Build history of the part. All positions in model axes, mm. Face numbers are marked on the shaded views. A direction names the side the tool comes from. Coordinates: 2 decimals unless noted, no trailing zeros. Write each loop counter-clockwise with the first axis right and the second up, starting at its lowest first coordinate (ties: lowest second). Pieces come first, ordered by that corner, then holes.
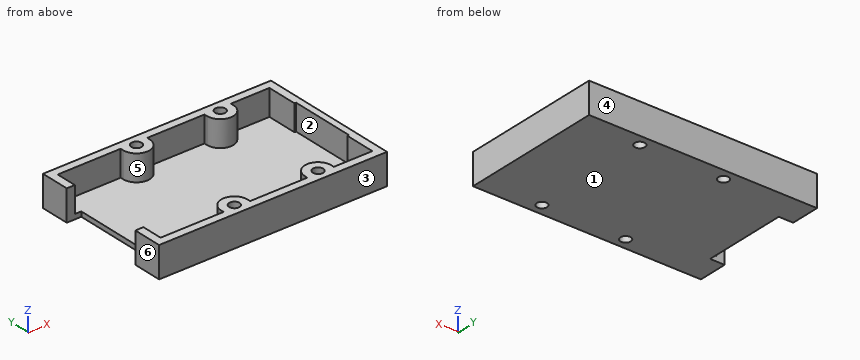
```python
from build123d import *

# Parameters (mm, degrees)
SKETCH_W                = 70.5
SKETCH_H                = 44
PAD_DEPTH               = 9.525
SKETCH001_R             = 1.6
POCKET_DEPTH            = 176.821853
SKETCH001_MIRRORED_2_R  = 1.6
POCKET_MIRRORED_2_DEPTH = 176.821853
POCKET001_DEPTH         = 8.025
SKETCH003_W             = 4.5
SKETCH003_H             = 26
POCKET002_DEPTH         = 9.526


with BuildPart() as part:
    # Sketch → Pad (new body)
    with BuildSketch(Plane.XY):
        with Locations((-3.8, 0)):
            Rectangle(SKETCH_W, SKETCH_H)
    extrude(amount=-PAD_DEPTH)

    # Sketch001 (on Face5 of Pad) → Pocket (cut, through all)
    with BuildSketch(Plane.XY):
        with Locations((-12.95, 18.55)):
            Circle(SKETCH001_R)
    pocket = extrude(amount=-POCKET_DEPTH, mode=Mode.SUBTRACT)

    # Sketch001 Mirrored 2 → Pocket Mirrored 2 (cut, through all)
    with BuildSketch(Plane(origin=(0, 0, 0), x_dir=(-1, 0, 0), z_dir=(0, 0, -1))):
        with Locations((-12.95, 18.55)):
            Circle(SKETCH001_MIRRORED_2_R)
    pocket_mirrored_2 = extrude(amount=POCKET_MIRRORED_2_DEPTH, mode=Mode.SUBTRACT)

    # Mirrored001: Pocket, Pocket Mirrored 2 across XZ
    add(pocket.mirror(Plane.XZ), mode=Mode.SUBTRACT)
    add(pocket_mirrored_2.mirror(Plane.XZ), mode=Mode.SUBTRACT)

    # Sketch002 (on Face4 of MultiTransform) → Pocket001 (cut)
    with BuildSketch(Plane.XY):
        with BuildLine():
            Line((29.45, -10), (29.45, 10))
            Line((29.45, 10), (28.95, 10))
            Line((28.95, 10), (28.95, 19.5))
            Line((28.95, 19.5), (17.05, 19.5))
            Line((17.05, 19.5), (17.05, 18.55))
            ThreePointArc((8.85, 18.55), (12.95, 14.45), (17.05, 18.55))
            Line((8.85, 19.5), (8.85, 18.55))
            Line((8.85, 19.5), (-8.85, 19.5))
            Line((-8.85, 19.5), (-8.85, 18.55))
            ThreePointArc((-17.05, 18.55), (-12.95, 14.45), (-8.85, 18.55))
            Line((-17.05, 19.5), (-17.05, 18.55))
            Line((-17.05, 19.5), (-36.55, 19.5))
            Line((-36.55, 19.5), (-36.55, -19.5))
            Line((-36.55, -19.5), (-17.05, -19.5))
            Line((-17.05, -19.5), (-17.05, -18.549995))
            ThreePointArc((-8.85, -18.549995), (-12.95, -14.45), (-17.05, -18.549995))
            Line((-8.85, -19.5), (-8.85, -18.549995))
            Line((8.85, -19.5), (-8.85, -19.5))
            Line((8.85, -19.5), (8.85, -18.549999))
            ThreePointArc((17.05, -18.55), (12.95, -14.45), (8.85, -18.549999))
            Line((17.05, -19.5), (17.05, -18.55))
            Line((17.05, -19.5), (28.95, -19.5))
            Line((28.95, -19.5), (28.95, -10))
            Line((28.95, -10), (29.45, -10))
        make_face()
    extrude(amount=-POCKET001_DEPTH, mode=Mode.SUBTRACT)

    # Sketch003 (on Face5 of Pocket001) → Pocket002 (cut, through all)
    with BuildSketch(Plane(origin=(0, 0, -9.525), x_dir=(1, 0, 0), z_dir=(0, 0, -1))):
        with Locations((-36.8, 0)):
            Rectangle(SKETCH003_W, SKETCH003_H)
    extrude(amount=-POCKET002_DEPTH, mode=Mode.SUBTRACT)


solid = part.part
```
1. 3-axis set-ups, long thin cutter, end or side, ignore diameter. For the marked faces 5 and 6: which of +Z, -Z, +X, -X, +Y, -Y reach the whole face in a straight line?
Computed values:
face 5: +Z
face 6: +Z, -Z, -X, +Y, -Y
2. Probe line 1 along Y through (x, z) = (-12.95, -6.5); line 2 along Y through (x, z) = (-34.5, -2.5); line 3 along Z through (x, y) = (-26, 7.5) (3 decimals). List the from-to ranges inside material, lowest first.
Computed values:
line 1: y = -22 to -20.15, -16.95 to -14.45, 14.45 to 16.95, 20.15 to 22
line 2: y = -22 to -19.5, 19.5 to 22
line 3: z = -9.525 to -8.025
3. Saw through at A-A on x = -12.95. List the corners of the cut face in (y, z) (3 decimals).
Computed values:
outline: (-22, -9.525) - (-20.15, -9.525) - (-20.15, 0) - (-22, 0) - close; (-16.95, -9.525) - (16.95, -9.525) - (16.95, 0) - (14.45, 0) - (14.45, -8.025) - (-14.45, -8.025) - (-14.45, 0) - (-16.95, 0) - close; (20.15, -9.525) - (22, -9.525) - (22, 0) - (20.15, 0) - close
4. Saw through at B-B on y = 12. List the corners of the cut face in (x, z) (3 decimals), plus the area to 3 significant figures.
Computed values:
outline: (-34.55, -9.525) - (31.45, -9.525) - (31.45, 0) - (28.95, 0) - (28.95, -8.025) - (-34.55, -8.025) - close
area: 119 mm2
5. Mould opens along Y. For the marked faces 1, 2, 3 and 4 say: +Y half, -Y half, draft (parallel to the pull), parting line (faces both ways), or undercut.
Computed values:
face 1: draft
face 2: undercut
face 3: -Y half
face 4: +Y half
6. Saw through at C-C on x = -30.5. List the corners of the cut face in (y, z) (3 decimals), plus the area to 3 significant figures.
Computed values:
outline: (-22, -9.525) - (22, -9.525) - (22, 0) - (19.5, 0) - (19.5, -8.025) - (-19.5, -8.025) - (-19.5, 0) - (-22, 0) - close
area: 106 mm2
7. Saw through at D-D on z = -6.5. State how many separate pieces and enclosed holes the cut face has, plus the area to 3 significant figures.
Computed values:
separate pieces: 1
enclosed holes: 4
area: 577 mm2
8. Flat gauge pins, fed straight in: pin 1 (3.5 mm diameter, centred on x = -12.95, y = -18.55, fed in from -Z) (3 decimals); pin 2 (4 mm diameter, centred on y = 3.5, z = -5, fed in from -X); pin 3 (11.5 mm diameter, centred on x = -8, y = 0, fed in from +Z) (3 decimals). Where does each tip first touch, or does it go through?
Computed values:
pin 1: stops at z = -9.525
pin 2: stops at x = 29.45
pin 3: stops at z = -8.025
